Geometry check sheet. Reference: the model listing, model coordinates, mm. Round coordinates to 2 decimals unless told otherwise and drop trailing zeros. Write each loop counter-clockwise with the first axis right and the second up, starting at its lowest first coordinate (ties: lowest second). Pieces come first, ordered by that corner, then holes. Notation, with made-up numbers: (61, 27.5) -> (66, 27.5) arc R28 cw to (66, 52.5) -> close; hole circle Ø11 at (29, -25). An arc over 180 degrees is marked (long way). Use a Markdown table: item, result.
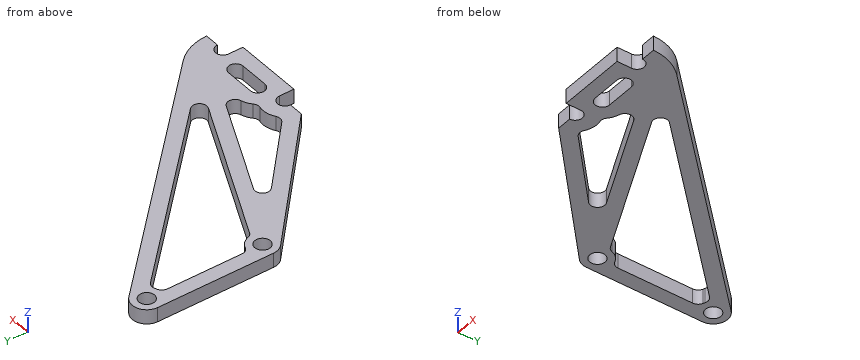
Autodesk Inventor part; units mm, degrees
ref_plane "YZ Plane" through (0, 0, 0) normal (1, 0, 0) x (0, 1, 0)
ref_plane "XZ Plane" through (0, 0, 0) normal (0, 1, 0) x (-1, 0, 0)
ref_plane "XY Plane" through (0, 0, 0) normal (0, 0, 1) x (1, 0, 0)
sketch "スケッチ1" plane through (0, 0, 0) normal (0, 0, 1) x (1, 0, 0)
  circle A0 centre (0, 0) radius 1.6
  arc A1 (2.1289, 2.1137) -> (-3, 0) centre (0, 0) ccw
  line L0 (43.813, -50.0351) -> (43.8106, -53.0351)
  line L1 (29.813, -50.0239) -> (29.8106, -53.0239)
  line L2 (46.9094, -42.9894) -> (2.1289, 2.1137)
  arc A2 (49.813, -50.0351) -> (46.9094, -42.9894) centre (39.813, -50.0351) ccw
  line L3 (49.813, -50.0351) -> (49.813, -50.0351)
  line L4 (49.813, -50.0351) -> (46.813, -50.0351)
  arc A3 (46.813, -50.0351) -> (43.813, -50.0351) centre (45.313, -50.0363) ccw
  line L5 (43.8106, -53.0351) -> (29.8106, -53.0239)
  arc A4 (29.813, -50.0239) -> (26.8131, -50.0351) centre (28.313, -50.0227) ccw
  line L6 (39.8106, -48.5351) -> (33.8106, -48.5351) construction
  line L7 (39.8106, -47.0351) -> (33.8106, -47.0351)
  line L8 (33.8106, -50.0351) -> (39.8106, -50.0351)
  arc A5 (39.8106, -50.0351) -> (39.8106, -47.0351) centre (39.8106, -48.5351) ccw
  arc A6 (33.8106, -47.0351) -> (33.8106, -50.0351) centre (33.8106, -48.5351) ccw
  line L9 (23.8131, -50.0351) -> (26.8131, -50.0351)
  circle A7 centre (0, -24) radius 1.6
  arc A8 (-3, -24) -> (-2.0335, -26.2056) centre (0, -24) ccw
  line L10 (-3, -24) -> (-3, 0)
  line L11 (-2.0335, -26.2056) -> (23.8131, -50.0351)
  point P0 (36.8106, -53.0295)
  point P1 (36.8106, -48.5351)
  point P2 (36.8106, -50.0351)
  dimension "d0" = 3.2
  dimension "d1" = 6
  dimension "d4" = 1.5
  dimension "d5" = 3
  dimension "d8" = 6
  dimension "d9" = 1.5
  dimension "d10" = 3
  dimension "d13" = 10
  dimension "d14" = 3.2
  dimension "d15" = 24
extrude "押し出し1" add sketch "スケッチ1" along normal blind 3
sketch "スケッチ2" plane through (0, 0, 3) normal (0, 0, 1) x (1, 0, 0)
  arc A0 (39.8106, -50.0351) -> (39.8106, -47.0351) centre (39.8106, -48.5351) ccw
  line L0 (39.8106, -50.0351) -> (33.8106, -50.0351)
  arc A1 (33.8106, -47.0351) -> (33.8106, -50.0351) centre (33.8106, -48.5351) ccw
  line L1 (33.8106, -47.0351) -> (39.8106, -47.0351)
  circle A2 centre (0, -24) radius 1.6
  circle A3 centre (0, 0) radius 1.6
  arc A4 (46.813, -50.0351) -> (43.813, -50.0351) centre (45.313, -50.0363) ccw
  line L2 (46.813, -50.0351) -> (49.813, -50.0351)
  arc A5 (49.813, -50.0351) -> (46.9094, -42.9894) centre (39.813, -50.0351) ccw
  line L3 (46.9094, -42.9894) -> (2.1289, 2.1137)
  arc A6 (2.1289, 2.1137) -> (-3, 0) centre (0, 0) ccw
  line L4 (-3, 0) -> (-3, -24)
  arc A7 (-3, -24) -> (-2.0335, -26.2056) centre (0, -24) ccw
  line L5 (-2.0335, -26.2056) -> (23.8131, -50.0351)
  line L6 (23.8131, -50.0351) -> (26.8131, -50.0351)
  arc A8 (29.813, -50.0239) -> (26.8131, -50.0351) centre (28.313, -50.0227) ccw
  line L7 (29.813, -50.0239) -> (29.8106, -53.0239)
  line L8 (29.8106, -53.0239) -> (43.8106, -53.0351)
  line L9 (43.8106, -53.0351) -> (43.813, -50.0351)
  arc A9 (45.1777, -45.5383) -> (44.7805, -45.1031) centre (39.813, -50.0351) ccw
  arc A10 (45.1777, -45.5383) -> (40.813, -50.0327) centre (45.313, -50.0363) ccw
  line L10 (40.813, -50.0327) -> (32.813, -50.0263)
  arc A11 (39.8106, -53.0351) -> (43.4781, -45.9274) centre (39.8106, -48.5351) ccw
  line L11 (39.8106, -53.0351) -> (33.8106, -53.0351)
  line L12 (33.8106, -44.0351) -> (38.5389, -44.0351)
  line L13 (0, -24) -> (45.1777, -45.5383) construction
  arc A12 (0, -22.5) -> (-0.6455, -25.354) centre (0, -24) ccw
  arc A13 (44.5321, -46.8923) -> (45.8232, -44.1843) centre (45.1777, -45.5383) ccw
  line L14 (43.0134, -46.1682) -> (44.5321, -46.8923)
  arc A14 (32.813, -50.0263) -> (32.3777, -48.0917) centre (28.313, -50.0227) ccw
  arc A15 (30.1517, -45.9155) -> (24.9646, -47.0163) centre (28.313, -50.0227) ccw
  arc A16 (33.8106, -44.0351) -> (30.1517, -45.9155) centre (33.8106, -48.5351) ccw
  arc A17 (29.3269, -48.9172) -> (33.8106, -53.0351) centre (33.8106, -48.5351) ccw
  line L15 (0, 0) -> (1.1273, -1.1354)
  line L16 (2.1137, -2.1289) -> (42.1113, -42.4147)
  line L17 (0, -1.6) -> (0, 0)
  arc A18 (2.1289, 2.1137) -> (-3, 0) centre (0, 0) ccw
  arc A19 (0, -3) -> (2.1137, -2.1289) centre (0, 0) ccw
  line L18 (-0.6455, -25.354) -> (1.6997, -26.4721)
  line L19 (3.7325, -27.4412) -> (38.5389, -44.0351)
  line L20 (24.9646, -47.0163) -> (3.7325, -27.4412)
  line L21 (2.2056, -26.0335) -> (0, -24)
  line L22 (42.1113, -42.4147) -> (2.9907, -23.7641)
  line L23 (1.1481, -22.8856) -> (0.6455, -22.646)
  line L24 (0, -24) -> (0, -22.4)
  line L25 (0, -21) -> (0, -3)
  arc A20 (2.9907, -23.7641) -> (0, -21) centre (0, -24) ccw
  arc A21 (-3, -24) -> (2.2056, -26.0335) centre (0, -24) ccw
  point P0 (22.5888, -34.7692)
  dimension "d17" = 3
  dimension "d18" = 3
extrude "押し出し2" cut sketch "スケッチ2" against normal blind 3 contours A16 A15 L20 L19 L12 | L16 L22 A20 L25 A19
fillet "フィレット1" radius 1.5 9 edges at (24.9646, -47.0163, 1.5) (30.1517, -45.9155, 1.5) (38.5389, -44.0351, 1.5) (3.7325, -27.4412, 1.5) (0, -21, 1.5) (2.9907, -23.7641, 1.5) (0, -3, 1.5) (2.1137, -2.1289, 1.5) (42.1113, -42.4147, 1.5)
properties part number "Tens1"
(1) Thickness scan on line 1 (Y direction, x = 30, z = 1.95); line 2 (X direction, y = -35, z = 1.5); line 3 (Y direction, x = 5.5, z = 0.4). Record the ranges inside material, lowest first.
A:
| item | result |
|---|---|
| line 1 | y = -53.02 to -45.65, -39.96 to -36.64, -30.22 to -25.96 |
| line 2 | x = 7.51 to 11.93, 19.59 to 26.56, 34.75 to 38.98 |
| line 3 | y = -33.15 to -24.96, -5.54 to -1.28 |
(2) Gauge pin test, flat ends, axial feed: pin 1 Ø1 at (y, z) = (-8.5, 1.5) entering from +X; pin 2 Ø10 at (x, y) = (5.5, -24) entering from -Z; pin 3 Ø1.9 at (x, y) = (0, 0) entering from +Z; pin 4 Ø1 at (y, z) = (-44, 1) entering from +X. Record the tip position at first contact, or that the pin passes through.
A:
| item | result |
|---|---|
| pin 1 | stops at x = 13.16 |
| pin 2 | stops at z = 0 |
| pin 3 | passes through |
| pin 4 | stops at x = 48.14 |
(3) Section check C-C on y = -35.5. Record the cut outline in (x, z).
A:
| item | result |
|---|---|
| outline | (8.05, 0) -> (12.47, 0) -> (12.47, 3) -> (8.05, 3) -> close; (20.64, 0) -> (27.61, 0) -> (27.61, 3) -> (20.64, 3) -> close; (35.25, 0) -> (39.47, 0) -> (39.47, 3) -> (35.25, 3) -> close |
(4) Section check A-A on y = -29. Record the cut outline in (x, z), plus the area to 3 significant figures.
A:
| item | result |
|---|---|
| outline | (1, 0) -> (13.97, 0) -> (13.97, 3) -> (1, 3) -> close; (28.79, 0) -> (33.02, 0) -> (33.02, 3) -> (28.79, 3) -> close |
| area | 51.6 mm2 |
(5) Section check B-B on x = 12. Record the cut outline in (y, z), plus the area to 3 significant figures.
A:
| item | result |
|---|---|
| outline | (-39.14, 0) -> (-35.06, 0) -> (-35.06, 3) -> (-39.14, 3) -> close; (-31.57, 0) -> (-28.06, 0) -> (-28.06, 3) -> (-31.57, 3) -> close; (-12.09, 0) -> (-7.83, 0) -> (-7.83, 3) -> (-12.09, 3) -> close |
| area | 35.5 mm2 |
(6) Section check D-D on y = -9. Record the cut outline in (x, z), plus the area to 3 significant figures.
A:
| item | result |
|---|---|
| outline | (-3, 0) -> (0, 0) -> (0, 3) -> (-3, 3) -> close; (8.94, 0) -> (13.16, 0) -> (13.16, 3) -> (8.94, 3) -> close |
| area | 21.7 mm2 |
